Could you check a few things on this model? Use its own coordinates, in mm. Round coordinates to 2 decimals unless told otherwise and drop trailing zeros. Loops run counter-clockwise (first coordinate to the right, second up) from the corner with the lowest first, then second, coordinate; pieces in that order, holes last. Notation, with made-up numbers: M 22.5,88.25 L 61.5,88.25 A35 ccw 61.5,127.25 Z; hole C 45.25,32 d2. An arc over 180 degrees is marked long. One line per item, written item: value. Start each with the question number.
Q1. Imagine slicing it at A-A (x = 0). Please give me the cut outline in (y, z) (1 decimal), then the cut area to 3 significant figures.
Q2. Please list where these lines run through material, in increasing order: line 1 along X through (y, z) = (0.4, 7); line 2 along X through (y, z) = (1.5, 6.75); line 3 along Z through (x, y) = (0, 0.8) (3 decimals).
Q3. Thinking about a two-plate mould opening in Z: for faces 1 (the face through (-2, 0, 0)), 2 (the face through (86.01, 0.78, 4.75)), which applies, released by +Z, released by -Z, zero draft, split by the parting line, or undercut?
Q4. I'm going to push a flat-ended pin straight in: pin 1 Ø3 at (x, z) = (97.31, 6.03) entering from -Y. Where does the tip first touch, or does it pass through?
from build123d import *

# Parameters (mm, degrees)
SKETCH2_W             = 215.9
SKETCH2_H             = 19.05
BOSS_EXTRUDE1_DEPTH   = 1.5875
F_6_CLEARANCE_HOLE1_D = 3.7973


with BuildPart() as part:
    # Sketch2 → Boss-Extrude1 (new body)
    with BuildSketch(Plane(origin=(0, 0, 0), x_dir=(1, 0, 0), z_dir=(0, 1, 0))):
        Rectangle(SKETCH2_W, SKETCH2_H)
    extrude(amount=BOSS_EXTRUDE1_DEPTH)

    # #6 Clearance Hole1 (through all)
    with Locations(Plane(origin=(0, 1.5875, 0), x_dir=(1, 0, 0), z_dir=(0, 1, 0))):
        with Locations((-97.31223666, -6.034928337), (0, -6.034928337), (97.31223666, -6.034928337), (-84.61223666, -6.034928337), (84.61223666, -6.034928337)):
            Hole(F_6_CLEARANCE_HOLE1_D / 2)


solid = part.part
Report:
1. outline: M 0,-9.5 L 1.6,-9.5 L 1.6,4.1 L 0,4.1 Z; M 0,7.9 L 1.6,7.9 L 1.6,9.5 L 0,9.5 Z
1. area: 24.2 mm²
2. line 1: x = -107.95 to -98.95, -95.68 to -86.25, -82.98 to -1.64, 1.64 to 82.98, 86.25 to 95.68, 98.95 to 107.95
2. line 2: x = -107.95 to -99.07, -95.55 to -86.37, -82.85 to -1.76, 1.76 to 82.85, 86.37 to 95.55, 99.07 to 107.95
2. line 3: z = -9.525 to 4.136, 7.934 to 9.525
3. face 1: zero draft
3. face 2: undercut
4. pin 1: passes through
